CAD build for the part. Positions are in the model's coordinates, mm. Face numbers are marked on the shaded views. A direction names the side the tool comes from. Coordinates: 2 decimals unless noted, no trailing zeros. Order: outer loops, then holes, each group sorted by start corner. A loop starts at its lowest first (then second) coordinate and runs counter-clockwise, first axis right, second up. Notation, with made-up numbers: (9.25, -7) - (32.25, -7) arc R20 cw to (32.25, 16) - close; hole circle Ø3 at (19, 3.5). An arc over 180 degrees is marked (long way). Use one line per item in the form item = value.
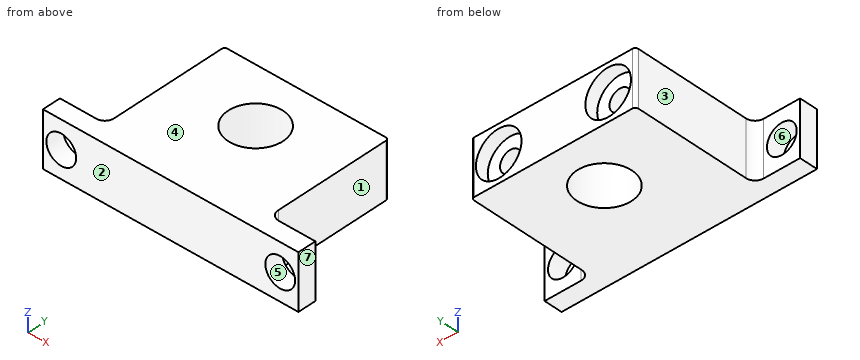
```python
from build123d import *

# Parameters (mm, degrees)
SKETCH1_R                                           = 4.7625
BOSS_EXTRUDE2_DEPTH                                 = 9.525
CBORE_FOR_6_BINDING_HEAD_MACHINE_SCREW1_D           = 3.6576
CBORE_FOR_6_BINDING_HEAD_MACHINE_SCREW1_DEPTH       = 14.224
CBORE_FOR_6_BINDING_HEAD_MACHINE_SCREW1_CBORE_D     = 7.9375
CBORE_FOR_6_BINDING_HEAD_MACHINE_SCREW1_CBORE_DEPTH = 2.2098
CBORE_FOR_6_BINDING_HEAD_MACHINE_SCREW1_TIP         = 1.0988539
F_6_0_204_DIAMETER_HOLE1_D                          = 5.1816


with BuildPart() as part:
    # Sketch1 → Boss-Extrude2 (new body)
    with BuildSketch(Plane.XY):
        with BuildLine():
            Line((22.225, -12.7), (-22.225, -12.7))
            Line((-22.225, -12.7), (-22.225, -9.535669584))
            Line((-22.225, -9.535669584), (-15.875, -9.535669584))
            ThreePointArc((-15.875, -9.535669584), (-14.752467985, -9.070701599), (-14.2875, -7.948169584))
            Line((-14.2875, -7.948169584), (-14.2875, 3.175))
            Line((-14.2875, 3.175), (-14.2875, 12.192))
            ThreePointArc((-14.2875, 12.192), (-14.138710245, 12.551210245), (-13.7795, 12.7))
            Line((-13.7795, 12.7), (13.7795, 12.7))
            ThreePointArc((13.7795, 12.7), (14.138710245, 12.551210245), (14.2875, 12.192))
            Line((14.2875, 12.192), (14.2875, 3.175))
            Line((14.2875, 3.175), (14.2875, -7.934401915))
            ThreePointArc((14.2875, -7.934401915), (14.756500442, -9.066669142), (15.888767669, -9.535669584))
            Line((15.888767669, -9.535669584), (22.225, -9.535669584))
            Line((22.225, -9.535669584), (22.225, -12.7))
        make_face()
        with Locations(Location((0, 3.175, 0), (0, 0, 180))):
            Circle(SKETCH1_R, mode=Mode.SUBTRACT)
    extrude(amount=BOSS_EXTRUDE2_DEPTH)

    # CBORE for #6 Binding Head Machine Screw1
    with Locations(Plane(origin=(0, 12.7, 0), x_dir=(1, 0, 0), z_dir=(0, 1, 0))):
        with Locations((9.525, -4.7625), (-9.525, -4.7625)):
            CounterBoreHole(CBORE_FOR_6_BINDING_HEAD_MACHINE_SCREW1_D / 2, CBORE_FOR_6_BINDING_HEAD_MACHINE_SCREW1_CBORE_D / 2, CBORE_FOR_6_BINDING_HEAD_MACHINE_SCREW1_CBORE_DEPTH, depth=CBORE_FOR_6_BINDING_HEAD_MACHINE_SCREW1_DEPTH)
            with Locations((0, 0, -(CBORE_FOR_6_BINDING_HEAD_MACHINE_SCREW1_DEPTH + CBORE_FOR_6_BINDING_HEAD_MACHINE_SCREW1_TIP / 2))):  # 118° drill point
                Cone(0, CBORE_FOR_6_BINDING_HEAD_MACHINE_SCREW1_D / 2, CBORE_FOR_6_BINDING_HEAD_MACHINE_SCREW1_TIP, mode=Mode.SUBTRACT)

    # #6 (0.204) Diameter Hole1 (through all)
    with Locations(Plane(origin=(0, -9.535669584, 0), x_dir=(1, 0, 0), z_dir=(0, 1, 0))):
        with Locations((-19.05, -4.699018138), (19.05, -4.699018138)):
            Hole(F_6_0_204_DIAMETER_HOLE1_D / 2)


solid = part.part
```
Item 1: 3-axis set-ups, long thin cutter, end or side, ignore diameter. For the marked faces 1, 2 and 3: which of +Z, -Z, +X, -X, +Y, -Y reach the whole face in a straight line?
Derived:
face_1 = +Z, -Z, +X, +Y
face_2 = +Z, -Z, +X, -X, -Y
face_3 = +Z, -Z, -X, +Y
Item 2: Cut at A-A, the plane x = 0. Write the cut outline in (y, z) (1 decimal), plus the area to 3 significant figures.
Derived:
outline = (-12.7, 0) - (-1.6, 0) - (-1.6, 9.5) - (-12.7, 9.5) - close; (7.9, 0) - (12.7, 0) - (12.7, 9.5) - (7.9, 9.5) - close
area = 151 mm²
Item 3: Drill centre lines: line 1 (Y direction, x = 0, z = 5.5); line 2 (X direction, y = -1, z = 5); line 3 (X direction, y = 9.25, z = 5). Where is each one in solid material? Low to high. Write a range as [from, to].
Derived:
line_1 = [-12.7, -1.59], [7.94, 12.7]
line_2 = [-14.29, -11.34], [-7.71, -2.29], [2.29, 7.71], [11.34, 14.29]
line_3 = [-14.29, -11.34], [-7.71, 7.71], [11.34, 14.29]
Item 4: Cut at C-C, the plane z = 4. State how many separate pieces and enclosed holes the cut face has, plus the area to 3 significant figures.
Derived:
separate_pieces = 3
enclosed_holes = 1
area = 557 mm²
Item 5: Drop flat-ended pins along their axis: pin 1 (4.5 mm diameter, centred on x = -19.05, z = 4.7, fed in from -Y); pin 2 (1 mm diameter, centred on y = -1, z = 8.5, fed in from -X); pin 3 (3 mm diameter, centred on y = 5.5, z = 4, fed in from +X); pin 4 (1.9 mm diameter, centred on x = -18, z = 7, fed in from +Y). Give the stop position or say it passes through.
Derived:
pin_1 = through
pin_2 = -14.29
pin_3 = 14.29
pin_4 = -9.54
Item 6: Two-plate mould, pull along Z, no slides. Class the marked faces 4, 5, 6 and 7: +Z half, -Z half, draft (parallel to the pull), parting line (faces both ways), or undercut.
Derived:
face_4 = +Z half
face_5 = undercut
face_6 = undercut
face_7 = draft
Item 7: Cut at D-D, the plane x = 19.05. Write the cut outline in (y, z) (3 decimals).
Derived:
outline = (-12.7, 0) - (-9.536, 0) - (-9.536, 2.108) - (-12.7, 2.108) - close; (-12.7, 7.29) - (-9.536, 7.29) - (-9.536, 9.525) - (-12.7, 9.525) - close
Item 8: Cut at B-B, the plane z = 8.25. Write the cut outline in (x, y) (1 decimal), plus the area to 3 significant figures.
Derived:
outline = (-22.2, -12.7) - (22.2, -12.7) - (22.2, -9.5) - (15.9, -9.5) arc R1.6 cw to (14.3, -7.9) - (14.3, 12.2) arc R0.5 ccw to (13.8, 12.7) - (11.4, 12.7) - (11.4, 10.5) - (7.6, 10.5) - (7.6, 12.7) - (-7.6, 12.7) - (-7.6, 10.5) - (-11.4, 10.5) - (-11.4, 12.7) - (-13.8, 12.7) arc R0.5 ccw to (-14.3, 12.2) - (-14.3, -7.9) arc R1.6 cw to (-15.9, -9.5) - (-22.2, -9.5) - close; hole circle Ø9.5 at (0, 3.2)
area = 689 mm²
